Answer from the drawing. Dimensions are ordinates in mm from the lowest x, y and z of the part. Round coordinates to 2 decimals unless told otherwise and drop trailing zeros. Loops run counter-clockwise (first coordinate to the right, second up) from the corner with the lowest first, then second, coordinate; pieces in that order, holes last. Notation, with made-up numbers: (-16, 10.5) - (4, 10.5) arc R18 ccw to (4, 44.5) - close; hole circle Ø1 at (-35, 66.5). An arc over 180 degrees is marked (long way). Answer as CSV lines item,"result". Start each with the question number.
Q1. Section D-D on y = 11 is taken. Write down the section's boundary in (x, z).
Q2. Straight lines are drawn through the part: L1, parallel to Z at x = 1.15, y = 38.1 (1 decimal); L2, parallel to Z at x = 0.15, y = 22.5 (1 decimal); L3, parallel to Z at x = 1, y = 14.5. For each, find the intervals that lie inside material, in ascending order. Write a range as [from, to].
Q3. Section A-A on x = 0.95 is taken. Count the separate pieces of the cut face and the enclosed holes in it, then the cut area to 3 significant figures.
Q4. Section B-B on y = 5.5 is taken. Write down the section's boundary in (x, z).
Q5. Section C-C on z = 5 is taken. Write down the section's boundary in (x, y).
Q6. Each of these flat-tipped pins is pushed along its axis until it touches: pin 1 Ø2.5 at (y, z) = (6.35, 31.75) entering from +X; pin 2 Ø0.5 at (x, z) = (1, 9.5) entering from -Y (1 decimal); pin 3 Ø0.5 at (x, y) = (0.5, 34) entering from -Z. Where does it stop, or does it pass through?
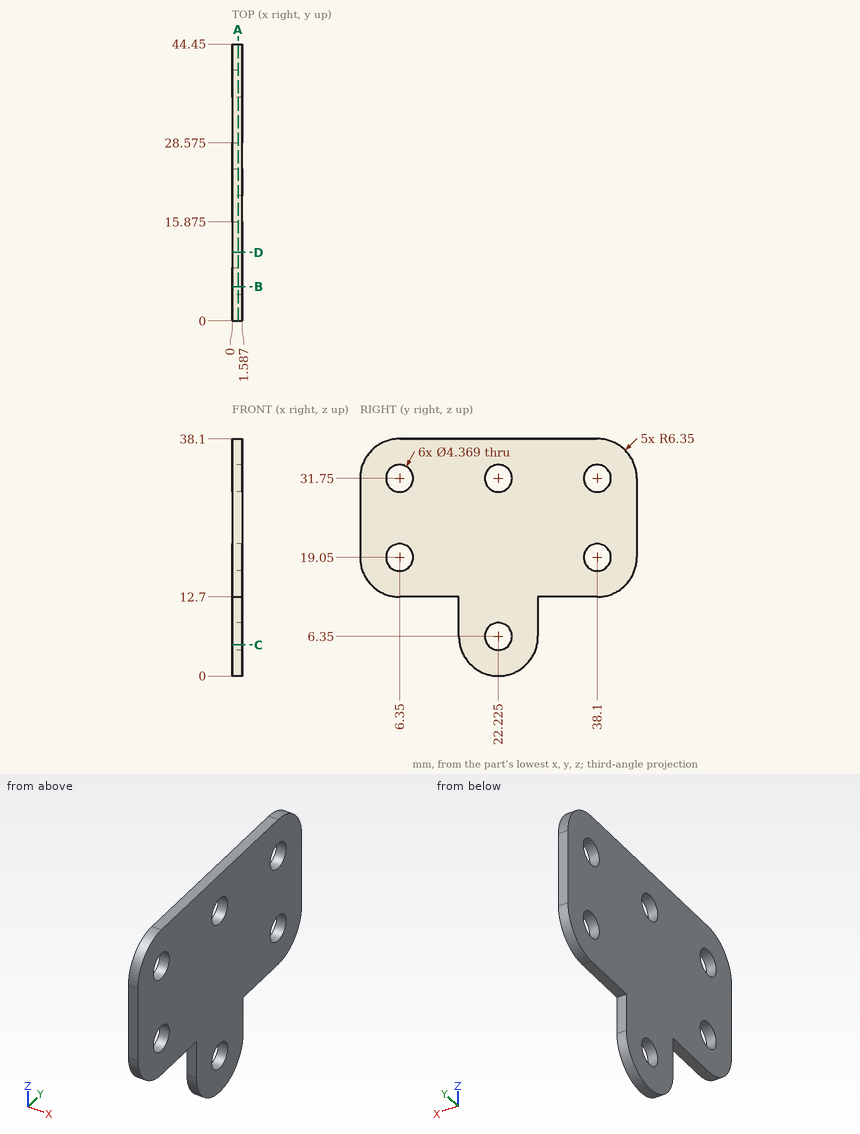
Findings:
1,outline,"(0, 12.7) - (1.59, 12.7) - (1.59, 38.1) - (0, 38.1) - close"
2,L1,"z = [12.7, 16.9], [21.2, 29.6], [33.9, 38.1]"
2,L2,"z = [0, 4.2], [8.5, 29.6], [33.9, 38.1]"
2,L3,"z = [12.7, 38.1]"
3,separate pieces,"1"
3,enclosed holes,"6"
3,area,"1,150 mm^2"
4,outline,"(0, 12.76) - (1.59, 12.76) - (1.59, 17.04) - (0, 17.04) - close; (0, 21.06) - (1.59, 21.06) - (1.59, 29.74) - (0, 29.74) - close; (0, 33.76) - (1.59, 33.76) - (1.59, 38.04) - (0, 38.04) - close"
5,outline,"(0, 16.02) - (1.59, 16.02) - (1.59, 20.51) - (0, 20.51) - close; (0, 23.94) - (1.59, 23.94) - (1.59, 28.43) - (0, 28.43) - close"
6,pin 1,"passes through"
6,pin 2,"stops at y = 15.9"
6,pin 3,"stops at z = 12.7"
